Geometry: final body of the model. Coordinates: model frame, mm. Face numbers are marked on the shaded views. A direction names the side the tool comes from. Give positions to 0.01 mm unless a question says otherwise; leave off trailing zeros. Loops run counter-clockwise (first coordinate to the right, second up) from the corner with the lowest first, then second, coordinate; pieces in that order, holes last.
1. Section C-C, the plane x = 171.5. Output: boundary loops of the cut face in (y, z) (3 decimals), then the cut area to 3 significant figures.
2. Section B-B, the plane x = 23. Output: boundary loops of the cut face in (y, z).
3. Access query for the marked faces 1 and 2. Directions: +Z, -Z, +X, -X, +Y, -Y. A direction counts if a zero-diameter tool reaches every point of the face in a straight line with its end or side. Return the directions, or none.
4. Material intervals for line 1 along Y through (x, z) = (46.5, 178.5); line 2 along Z through (x, y) = (-30, -10.5); line 3 along Z through (x, y) = (5, 8.5), sorted ascending.
5. First-contact query: P1, Ø1.5, axis at x = 82, z = 82, coming from the -Y side; P2, Ø3, axis at x = 8.5, z = 98, coming from the +Y side; P3, Ø8, axis at x = 125, y = 7, coming from the -Z side. Flat tips, straight axial feed; report the tip coordinate or a pass-through.
6. Section A-A, the plane z = 56. Output: boundary loops of the cut face in (x, y), then the cut area to 3 significant figures.
7. Draft query along Z for the marked faces 3, 4 and 5. Return one class per face: +Z half, -Z half, draft (parallel to the pull), parting line (faces both ways), or undercut.
from build123d import *

# Parameters (mm, degrees)
EXTRUDE_1_DEPTH     = 5
EXTRUDE_2_DEPTH     = 15
CUT_EXTRUDE_1_DEPTH = 60
SKETCH_4_R          = 4
CUT_EXTRUDE_2_DEPTH = 60
EXTRUDE_3_DEPTH     = 15
SKETCH_6_W          = 72.003415158
SKETCH_6_H          = 5
EXTRUDE_4_DEPTH     = 13
EXTRUDE_5_DEPTH     = 20
EXTRUDE_6_DEPTH     = 72


with BuildPart() as part:
    # 草图1 → 凸台-拉伸1 (new body)
    with BuildSketch(Plane(origin=(0, 0, 0), x_dir=(1, 0, 0), z_dir=(0, 1, 0))):
        Polygon((-50, 10), (-10, 50), (176.666666667, 3.333333333), (190, -10), (190, -120), (120, -190), (10, -190), (-3.333333333, -176.666666667), align=None)
    extrude(amount=EXTRUDE_1_DEPTH)

    # 草图2 → 凸台-拉伸2 (add)
    with BuildSketch(Plane.XZ):
        Polygon((-50, -10), (-39.393398282, 0.606601718), (0.606601718, -39.393398282), (-10, -50), align=None)
    extrude(amount=EXTRUDE_2_DEPTH)

    # 草图3 → 切除-拉伸1 (cut)
    with BuildSketch(Plane(origin=(20, 0, -20), x_dir=(-0.7071067811865475, 0, -0.7071067811865476), z_dir=(0.7071067811865476, 0, -0.7071067811865475))):
        with BuildLine():
            Line((27.426406871, -7.5), (27.426406871, -15))
            Line((27.426406871, -15), (34.926406871, -15))
            ThreePointArc((34.926406871, -15), (29.623106012, -12.803300859), (27.426406871, -7.5))
        make_face()
    extrude(amount=-CUT_EXTRUDE_1_DEPTH, mode=Mode.SUBTRACT)

    # 草图4 → 切除-拉伸2 (cut)
    with BuildSketch(Plane(origin=(20, 0, -20), x_dir=(-0.7071067811865474, 0, -0.7071067811865477), z_dir=(0.7071067811865477, 0, -0.7071067811865474))):
        with Locations((34.926406871, -7.5)):
            Circle(SKETCH_4_R)
        with BuildLine():
            Line((34.926406871, -15), (42.426406871, -15))
            Line((42.426406871, -15), (42.426406871, -7.5))
            ThreePointArc((42.426406871, -7.5), (40.22970773, -12.803300859), (34.926406871, -15))
        make_face()
    extrude(amount=-CUT_EXTRUDE_2_DEPTH, mode=Mode.SUBTRACT)

    # 草图5 → 凸台-拉伸3 (add)
    with BuildSketch(Plane(origin=(0, 5, 0), x_dir=(1, 0, 0), z_dir=(0, 1, 0))):
        Polygon((-0.62444127, -175.132918043), (11.242640687, -187), (118.757359313, -187), (187, -118.757359313), (187, -11.242640687), (175.132918043, 0.62444127), (8.675243128, 42.238859999), (4.552137502, 46.361965624), (176.666666667, 3.333333333), (190, -10), (190, -120), (120, -190), (10, -190), (-3.333333333, -176.666666667), (-46.361965624, -4.552137502), (-42.238859999, -8.675243128), align=None)
    extrude(amount=EXTRUDE_3_DEPTH)

    # 草图6 → 凸台-拉伸4 (add, symmetric)
    with BuildSketch(Plane(origin=(-30, 0, -30), x_dir=(-0.7071067811865475, 0, 0.7071067811865476), z_dir=(-0.7071067811865476, 0, -0.7071067811865475))):
        with Locations((0, 2.5)):
            Rectangle(SKETCH_6_W, SKETCH_6_H)
    extrude(amount=EXTRUDE_4_DEPTH, both=True)

    # 草图7 → 凸台-拉伸5 (add)
    with BuildSketch(Plane(origin=(0, 20, 0), x_dir=(1, 0, 0), z_dir=(0, 1, 0))):
        Polygon((-42.238859999, -8.675243128), (-64.649439719, 13.735336592), (-63.235226156, 8.078482343), (-44.947752062, -10.208991752), align=None)
        Polygon((8.675243128, 42.238859999), (-13.735336592, 64.649439719), (-8.078482343, 63.235226156), (10.208991752, 44.947752062), align=None)
    extrude(amount=-EXTRUDE_5_DEPTH)

    # 草图8 → 凸台-拉伸6 (add)
    with BuildSketch(Plane(origin=(25.457051563, 0, -25.457051563), x_dir=(0.7071067811865439, 0, 0.7071067811865511), z_dir=(-0.7071067811865511, 0, 0.7071067811865439))):
        Polygon((-55.426406871, 20), (-23.733061091, 5), (-55.426406871, 5), align=None)
    extrude(amount=EXTRUDE_6_DEPTH)


solid = part.part
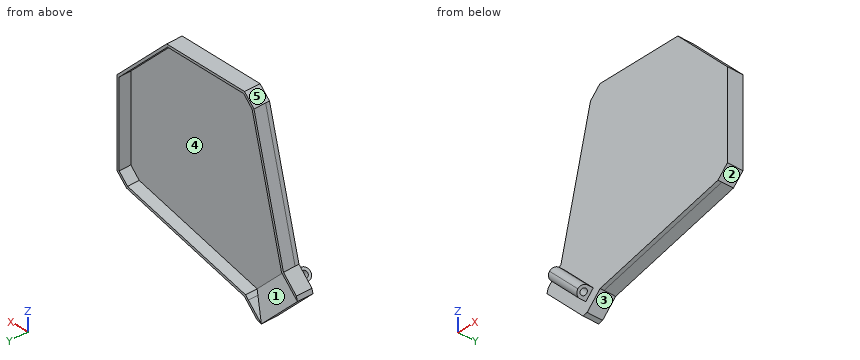
Answers below:
1. outline: (0, -4.625) - (20, -4.625) - (20, -1.533) - (5, -1.533) - (5, 134.257) - (20, 134.257) - (20, 138.5) - (0, 138.5) - close
1. area: 826 mm2
2. outline: (0, -41.75) - (20, -41.75) - (20, -38.66) - (5, -38.66) - (5, 187) - (20, 187) - (20, 190) - (0, 190) - close
3. face 1: +Y
3. face 2: -Z, +X, +Y, -Y
4. line 1: y = 0 to 5
4. line 2: z = -29.11 to -23.14, -15.65 to -9.67
4. line 3: z = -50.16 to -45.91, 180.76 to 185
5. P1: stops at y = 0
5. P2: stops at y = 5
5. P3: stops at z = -17.25
6. outline: (-33.5, 0) - (190, 0) - (190, 20) - (187, 20) - (187, 5) - (-30.41, 5) - (-30.41, 20) - (-33.5, 20) - close
6. area: 1,210 mm2
7. face 3: -Z half
7. face 4: undercut
7. face 5: +Z half
